Geometry check sheet. Reference: the model listing, model coordinates, mm. Face numbers are marked on the shaded views. A direction names the side the tool comes from. Round coordinates to 2 decimals unless told otherwise and drop trailing zeros. Loops run counter-clockwise (first coordinate to the right, second up) from the corner with the lowest first, then second, coordinate; pieces in that order, holes last. Notation, with made-up numbers: (50.25, 76.25) -> (98.25, 76.25) arc R30 cw to (98.25, 112.25) -> close; hole circle Ø6 at (34.25, 66.5). An arc over 180 degrees is marked (long way). Use one line per item in the form item = value.
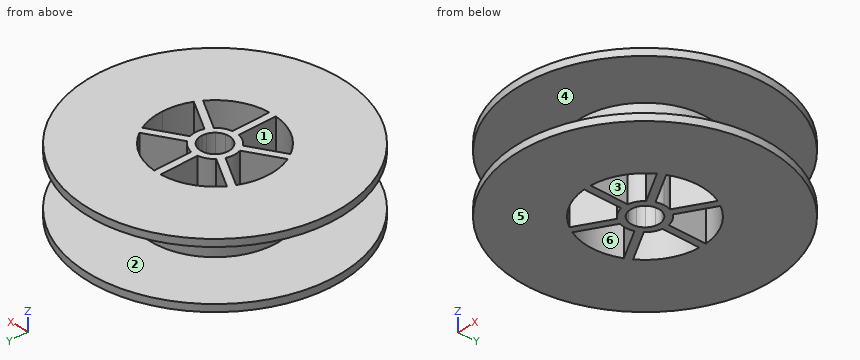
from build123d import *

# Parameters (mm, degrees)
F0_R     = 44.375
F1_DEPTH = 22.7
F2_R     = 44.375
F2_R_2   = 22.625
F3_DEPTH = 20.2
F4_R     = 44.375
F4_R_2   = 22.625
F5_DEPTH = 2.5


with BuildPart() as f1:
    # F0 (on Top) → F1 (new body)
    with BuildSketch(Plane.XY):
        Circle(F0_R)
        with BuildLine():
            ThreePointArc((18.0086459229, 8.9835570362), (19.5887674982, 4.6147386601), (20.125, 0))
            ThreePointArc((20.125, 0), (19.5887674982, -4.6147386601), (18.0086459229, -8.9835570362))
            Line((18.0086459229, -8.9835570362), (19.3430855029, -9.753996087))
            Line((19.3430855029, -9.753996087), (18.1187511512, -11.8746053896))
            Line((18.1187511512, -11.8746053896), (16.7843115712, -11.1041663389))
            ThreePointArc((16.7843115712, -11.1041663389), (10.0625, -17.4287612512), (1.2243343517, -20.0877233751))
            Line((1.2243343517, -20.0877233751), (1.2243343517, -21.6286014766))
            Line((1.2243343517, -21.6286014766), (-1.2243343517, -21.6286014766))
            Line((-1.2243343517, -21.6286014766), (-1.2243343517, -20.0877233751))
            ThreePointArc((-1.2243343517, -20.0877233751), (-10.0625, -17.4287612512), (-16.7843115712, -11.1041663389))
            Line((-16.7843115712, -11.1041663389), (-18.1187511512, -11.8746053896))
            Line((-18.1187511512, -11.8746053896), (-19.3430855029, -9.753996087))
            Line((-19.3430855029, -9.753996087), (-18.0086459229, -8.9835570362))
            ThreePointArc((-18.0086459229, -8.9835570362), (-20.125, 0), (-18.0086459229, 8.9835570362))
            Line((-18.0086459229, 8.9835570362), (-19.3430855029, 9.753996087))
            Line((-19.3430855029, 9.753996087), (-18.1187511512, 11.8746053896))
            Line((-18.1187511512, 11.8746053896), (-16.7843115712, 11.1041663389))
            ThreePointArc((-16.7843115712, 11.1041663389), (-10.0625, 17.4287612512), (-1.2243343517, 20.0877233751))
            Line((-1.2243343517, 20.0877233751), (-1.2243343517, 21.6286014766))
            Line((-1.2243343517, 21.6286014766), (1.2243343517, 21.6286014766))
            Line((1.2243343517, 21.6286014766), (1.2243343517, 20.0877233751))
            ThreePointArc((1.2243343517, 20.0877233751), (10.0625, 17.4287612512), (16.7843115712, 11.1041663389))
            Line((16.7843115712, 11.1041663389), (18.1187511512, 11.8746053896))
            Line((18.1187511512, 11.8746053896), (19.3430855029, 9.753996087))
            Line((19.3430855029, 9.753996087), (18.0086459229, 8.9835570362))
        make_face(mode=Mode.SUBTRACT)
        with BuildLine():
            Line((-5.5763406448, 4.6332413075), (-16.7843115712, 11.1041663389))
            ThreePointArc((-16.7843115712, 11.1041663389), (-17.4287612512, 10.0625), (-18.0086459229, 8.9835570362))
            Line((-18.0086459229, 8.9835570362), (-6.8006749965, 2.5126320048))
            ThreePointArc((-6.8006749965, 2.5126320048), (-6.2786841774, 3.625), (-5.5763406448, 4.6332413075))
        make_face()
        with BuildLine():
            Line((1.2243343517, 7.1458733123), (1.2243343517, 20.0877233751))
            ThreePointArc((1.2243343517, 20.0877233751), (0, 20.125), (-1.2243343517, 20.0877233751))
            Line((-1.2243343517, 20.0877233751), (-1.2243343517, 7.1458733123))
            ThreePointArc((-1.2243343517, 7.1458733123), (0, 7.25), (1.2243343517, 7.1458733123))
        make_face()
        with BuildLine():
            Line((6.8006749965, 2.5126320048), (18.0086459229, 8.9835570362))
            ThreePointArc((18.0086459229, 8.9835570362), (17.4287612512, 10.0625), (16.7843115712, 11.1041663389))
            Line((16.7843115712, 11.1041663389), (5.5763406448, 4.6332413075))
            ThreePointArc((5.5763406448, 4.6332413075), (6.2786841774, 3.625), (6.8006749965, 2.5126320048))
        make_face()
        with BuildLine():
            ThreePointArc((16.7843115712, -11.1041663389), (17.4287612512, -10.0625), (18.0086459229, -8.9835570362))
            Line((18.0086459229, -8.9835570362), (6.8006749965, -2.5126320048))
            ThreePointArc((6.8006749965, -2.5126320048), (6.2786841774, -3.625), (5.5763406448, -4.6332413075))
            Line((5.5763406448, -4.6332413075), (16.7843115712, -11.1041663389))
        make_face()
        with BuildLine():
            ThreePointArc((-18.0086459229, -8.9835570362), (-17.4287612512, -10.0625), (-16.7843115712, -11.1041663389))
            Line((-16.7843115712, -11.1041663389), (-5.5763406448, -4.6332413075))
            ThreePointArc((-5.5763406448, -4.6332413075), (-6.2786841774, -3.625), (-6.8006749965, -2.5126320048))
            Line((-6.8006749965, -2.5126320048), (-18.0086459229, -8.9835570362))
        make_face()
        with BuildLine():
            ThreePointArc((-1.2243343517, -20.0877233751), (0, -20.125), (1.2243343517, -20.0877233751))
            Line((1.2243343517, -20.0877233751), (1.2243343517, -7.1458733123))
            ThreePointArc((1.2243343517, -7.1458733123), (0, -7.25), (-1.2243343517, -7.1458733123))
            Line((-1.2243343517, -7.1458733123), (-1.2243343517, -20.0877233751))
        make_face()
        with BuildLine():
            ThreePointArc((-18.0086459229, 8.9835570362), (-17.4287612512, 10.0625), (-16.7843115712, 11.1041663389))
            Line((-16.7843115712, 11.1041663389), (-18.1187511512, 11.8746053896))
            Line((-18.1187511512, 11.8746053896), (-19.3430855029, 9.753996087))
            Line((-19.3430855029, 9.753996087), (-18.0086459229, 8.9835570362))
        make_face()
        with BuildLine():
            ThreePointArc((-1.2243343517, 20.0877233751), (0, 20.125), (1.2243343517, 20.0877233751))
            Line((1.2243343517, 20.0877233751), (1.2243343517, 21.6286014766))
            Line((1.2243343517, 21.6286014766), (-1.2243343517, 21.6286014766))
            Line((-1.2243343517, 21.6286014766), (-1.2243343517, 20.0877233751))
        make_face()
        with BuildLine():
            ThreePointArc((16.7843115712, 11.1041663389), (17.4287612512, 10.0625), (18.0086459229, 8.9835570362))
            Line((18.0086459229, 8.9835570362), (19.3430855029, 9.753996087))
            Line((19.3430855029, 9.753996087), (18.1187511512, 11.8746053896))
            Line((18.1187511512, 11.8746053896), (16.7843115712, 11.1041663389))
        make_face()
        with BuildLine():
            Line((19.3430855029, -9.753996087), (18.0086459229, -8.9835570362))
            ThreePointArc((18.0086459229, -8.9835570362), (17.4287612512, -10.0625), (16.7843115712, -11.1041663389))
            Line((16.7843115712, -11.1041663389), (18.1187511512, -11.8746053896))
            Line((18.1187511512, -11.8746053896), (19.3430855029, -9.753996087))
        make_face()
        with BuildLine():
            Line((1.2243343517, -21.6286014766), (1.2243343517, -20.0877233751))
            ThreePointArc((1.2243343517, -20.0877233751), (0, -20.125), (-1.2243343517, -20.0877233751))
            Line((-1.2243343517, -20.0877233751), (-1.2243343517, -21.6286014766))
            Line((-1.2243343517, -21.6286014766), (1.2243343517, -21.6286014766))
        make_face()
        with BuildLine():
            Line((-18.1187511512, -11.8746053896), (-16.7843115712, -11.1041663389))
            ThreePointArc((-16.7843115712, -11.1041663389), (-17.4287612512, -10.0625), (-18.0086459229, -8.9835570362))
            Line((-18.0086459229, -8.9835570362), (-19.3430855029, -9.753996087))
            Line((-19.3430855029, -9.753996087), (-18.1187511512, -11.8746053896))
        make_face()
        with BuildLine():
            Line((-3.5861365347, 3.4841964288), (-5.5763406448, 4.6332413075))
            ThreePointArc((-5.5763406448, 4.6332413075), (-6.2786841774, 3.625), (-6.8006749965, 2.5126320048))
            Line((-6.8006749965, 2.5126320048), (-4.8104708865, 1.3635871261))
            ThreePointArc((-4.8104708865, 1.3635871261), (-4.3301270189, 2.5), (-3.5861365347, 3.4841964288))
        make_face()
        with BuildLine():
            Line((-4.8104708865, 1.3635871261), (-6.8006749965, 2.5126320048))
            ThreePointArc((-6.8006749965, 2.5126320048), (-7.25, 0), (-6.8006749965, -2.5126320048))
            Line((-6.8006749965, -2.5126320048), (-4.8104708865, -1.3635871261))
            ThreePointArc((-4.8104708865, -1.3635871261), (-5, 0), (-4.8104708865, 1.3635871261))
        make_face()
        with BuildLine():
            ThreePointArc((-6.8006749965, -2.5126320048), (-6.2786841774, -3.625), (-5.5763406448, -4.6332413075))
            Line((-5.5763406448, -4.6332413075), (-3.5861365347, -3.4841964288))
            ThreePointArc((-3.5861365347, -3.4841964288), (-4.3301270189, -2.5), (-4.8104708865, -1.3635871261))
            Line((-4.8104708865, -1.3635871261), (-6.8006749965, -2.5126320048))
        make_face()
        with BuildLine():
            ThreePointArc((-5.5763406448, -4.6332413075), (-3.625, -6.2786841774), (-1.2243343517, -7.1458733123))
            Line((-1.2243343517, -7.1458733123), (-1.2243343517, -4.8477835549))
            ThreePointArc((-1.2243343517, -4.8477835549), (-2.5, -4.3301270189), (-3.5861365347, -3.4841964288))
            Line((-3.5861365347, -3.4841964288), (-5.5763406448, -4.6332413075))
        make_face()
        with BuildLine():
            ThreePointArc((-1.2243343517, -7.1458733123), (0, -7.25), (1.2243343517, -7.1458733123))
            Line((1.2243343517, -7.1458733123), (1.2243343517, -4.8477835549))
            ThreePointArc((1.2243343517, -4.8477835549), (0, -5), (-1.2243343517, -4.8477835549))
            Line((-1.2243343517, -4.8477835549), (-1.2243343517, -7.1458733123))
        make_face()
        with BuildLine():
            ThreePointArc((5.5763406448, -4.6332413075), (6.2786841774, -3.625), (6.8006749965, -2.5126320048))
            Line((6.8006749965, -2.5126320048), (4.8104708865, -1.3635871261))
            ThreePointArc((4.8104708865, -1.3635871261), (4.3301270189, -2.5), (3.5861365347, -3.4841964288))
            Line((3.5861365347, -3.4841964288), (5.5763406448, -4.6332413075))
        make_face()
        with BuildLine():
            ThreePointArc((7.25, 0), (7.1367847706, 1.2762457199), (6.8006749965, 2.5126320048))
            Line((6.8006749965, 2.5126320048), (4.8104708865, 1.3635871261))
            ThreePointArc((4.8104708865, 1.3635871261), (4.9523910605, 0.6883478654), (5, 0))
            ThreePointArc((5, 0), (4.9523910605, -0.6883478654), (4.8104708865, -1.3635871261))
            Line((4.8104708865, -1.3635871261), (6.8006749965, -2.5126320048))
            ThreePointArc((6.8006749965, -2.5126320048), (7.1367847706, -1.2762457199), (7.25, 0))
        make_face()
        with BuildLine():
            Line((4.8104708865, 1.3635871261), (6.8006749965, 2.5126320048))
            ThreePointArc((6.8006749965, 2.5126320048), (6.2786841774, 3.625), (5.5763406448, 4.6332413075))
            Line((5.5763406448, 4.6332413075), (3.5861365347, 3.4841964288))
            ThreePointArc((3.5861365347, 3.4841964288), (4.3301270189, 2.5), (4.8104708865, 1.3635871261))
        make_face()
        with BuildLine():
            Line((3.5861365347, 3.4841964288), (5.5763406448, 4.6332413075))
            ThreePointArc((5.5763406448, 4.6332413075), (3.625, 6.2786841774), (1.2243343517, 7.1458733123))
            Line((1.2243343517, 7.1458733123), (1.2243343517, 4.8477835549))
            ThreePointArc((1.2243343517, 4.8477835549), (2.5, 4.3301270189), (3.5861365347, 3.4841964288))
        make_face()
        with BuildLine():
            Line((-1.2243343517, 4.8477835549), (-1.2243343517, 7.1458733123))
            ThreePointArc((-1.2243343517, 7.1458733123), (-3.625, 6.2786841774), (-5.5763406448, 4.6332413075))
            Line((-5.5763406448, 4.6332413075), (-3.5861365347, 3.4841964288))
            ThreePointArc((-3.5861365347, 3.4841964288), (-2.5, 4.3301270189), (-1.2243343517, 4.8477835549))
        make_face()
        with BuildLine():
            Line((1.2243343517, 4.8477835549), (1.2243343517, 7.1458733123))
            ThreePointArc((1.2243343517, 7.1458733123), (0, 7.25), (-1.2243343517, 7.1458733123))
            Line((-1.2243343517, 7.1458733123), (-1.2243343517, 4.8477835549))
            ThreePointArc((-1.2243343517, 4.8477835549), (0, 5), (1.2243343517, 4.8477835549))
        make_face()
        with BuildLine():
            ThreePointArc((1.2243343517, -7.1458733123), (3.625, -6.2786841774), (5.5763406448, -4.6332413075))
            Line((5.5763406448, -4.6332413075), (3.5861365347, -3.4841964288))
            ThreePointArc((3.5861365347, -3.4841964288), (2.5, -4.3301270189), (1.2243343517, -4.8477835549))
            Line((1.2243343517, -4.8477835549), (1.2243343517, -7.1458733123))
        make_face()
    extrude(amount=F1_DEPTH)

    # F2 (on face) → F3 (cut)
    with BuildSketch(Plane.XY.offset(22.7)):
        Circle(F2_R)
        Circle(F2_R_2, mode=Mode.SUBTRACT)
    extrude(amount=-F3_DEPTH, mode=Mode.SUBTRACT)

    # F4 (on face) → F5 (join)
    with BuildSketch(Plane.XY.offset(22.7)):
        Circle(F4_R)
        Circle(F4_R_2, mode=Mode.SUBTRACT)
    extrude(amount=-F5_DEPTH)


solid = f1.part
1. Section check D-D (z = 7.25). Record the boundary of the cut face in (x, y) (3 decimals), then the cut area to 3 significant figures.
Return value:
outline = circle Ø45.25 at (0, 0); hole (-18.009, -8.984) -> (-6.801, -2.513) arc R7.25 cw to (-6.801, 2.513) -> (-18.009, 8.984) arc R20.125 ccw to start; hole (-16.784, -11.104) arc R20.125 ccw to (-1.224, -20.088) -> (-1.224, -7.146) arc R7.25 cw to (-5.576, -4.633) -> close; hole (-16.784, 11.104) -> (-5.576, 4.633) arc R7.25 cw to (-1.224, 7.146) -> (-1.224, 20.088) arc R20.125 ccw to start; hole circle Ø10 at (0, 0); hole (1.224, -20.088) arc R20.125 ccw to (16.784, -11.104) -> (5.576, -4.633) arc R7.25 cw to (1.224, -7.146) -> close; hole (1.224, 7.146) arc R7.25 cw to (5.576, 4.633) -> (16.784, 11.104) arc R20.125 ccw to (1.224, 20.088) -> close; hole (6.801, -2.513) -> (18.009, -8.984) arc R20.125 ccw to (18.009, 8.984) -> (6.801, 2.513) arc R7.25 cw to start
area = 612 mm2
2. Section check B-B (x = -9). Record the boundary of the cut face in (y, z), then the cut area to 3 significant figures.
Return value:
outline = (-43.45, 0) -> (-18, 0) -> (-18, 22.7) -> (-43.45, 22.7) -> (-43.45, 20.2) -> (-20.76, 20.2) -> (-20.76, 2.5) -> (-43.45, 2.5) -> close; (-6.61, 0) -> (-3.78, 0) -> (-3.78, 22.7) -> (-6.61, 22.7) -> close; (3.78, 0) -> (6.61, 0) -> (6.61, 22.7) -> (3.78, 22.7) -> close; (18, 0) -> (43.45, 0) -> (43.45, 2.5) -> (20.76, 2.5) -> (20.76, 20.2) -> (43.45, 20.2) -> (43.45, 22.7) -> (18, 22.7) -> close
area = 481 mm2
3. Section check C-C (y = -27.5). Record the boundary of the cut face in (x, z).
Return value:
outline = (-34.83, 0) -> (34.83, 0) -> (34.83, 2.5) -> (-34.83, 2.5) -> close; (-34.83, 20.2) -> (34.83, 20.2) -> (34.83, 22.7) -> (-34.83, 22.7) -> close
4. Gauge pin test, flat ends, axial feed: pin 1 (4 mm diameter, centred on y = 12.5, z = 16, fed in from -X); pin 2 (3 mm diameter, centred on y = 11.5, z = 10.5, fed in from -X); pin 3 (2 mm diameter, centred on y = 2.5, z = 11.5, fed in from -X). Record the tip position at first contact, or that the pin passes through.
Return value:
pin_1 = -20.04
pin_2 = -20.3
pin_3 = -22.58
5. Material ranges on line 1 along Y through (x, z) = (-9.5, 15.5); line 2 along Z through (x, y) = (-22.5, -9.5); line 3 along X through (y, z) = (14, 15), recorded low to high.
Return value:
line_1 = -20.53 to -17.74, -6.9 to -4.07, 4.07 to 6.9, 17.74 to 20.53
line_2 = 0 to 2.5, 20.2 to 22.7
line_3 = -17.77 to -14.46, -1.22 to 1.22, 14.46 to 17.77
6. Section check A-A (x = 0). Record the boundary of the cut face in (y, z) (3 decimals), then the cut area to 3 significant figures.
Return value:
outline = (-44.375, 0) -> (-5, 0) -> (-5, 22.7) -> (-44.375, 22.7) -> (-44.375, 20.2) -> (-22.625, 20.2) -> (-22.625, 2.5) -> (-44.375, 2.5) -> close; (5, 0) -> (44.375, 0) -> (44.375, 2.5) -> (22.625, 2.5) -> (22.625, 20.2) -> (44.375, 20.2) -> (44.375, 22.7) -> (5, 22.7) -> close
area = 1,020 mm2
7. Mould release check, pull along Y, two halves, no side actions. Record for the marked faces 1, 2 and 3: released by +Y, released by -Y, zero draft, split by the parting line, or undercut.
Return value:
face_1 = undercut
face_2 = zero draft
face_3 = undercut
8. Tool access check on the marked faces 4, 5 and 6. Record the directions out of +Z, -Z, +X, -X, +Y, -Y that give a thin tool (end or side, any length) a straight path to the whole face; none if there is none.
Return value:
face_4 = none
face_5 = -Z, +X, -X, +Y, -Y
face_6 = +Z, -Z
